Check sheet for the drawn part. Datum: minimum x, y, z corner. Units: mm. Round coordinates to 2 decimals unless told otherwise and drop trailing zeros. Order: outer loops, then holes, each group sorted by start corner. A loop starts at its lowest first (then second) coordinate and runs counter-clockwise, first axis right, second up.
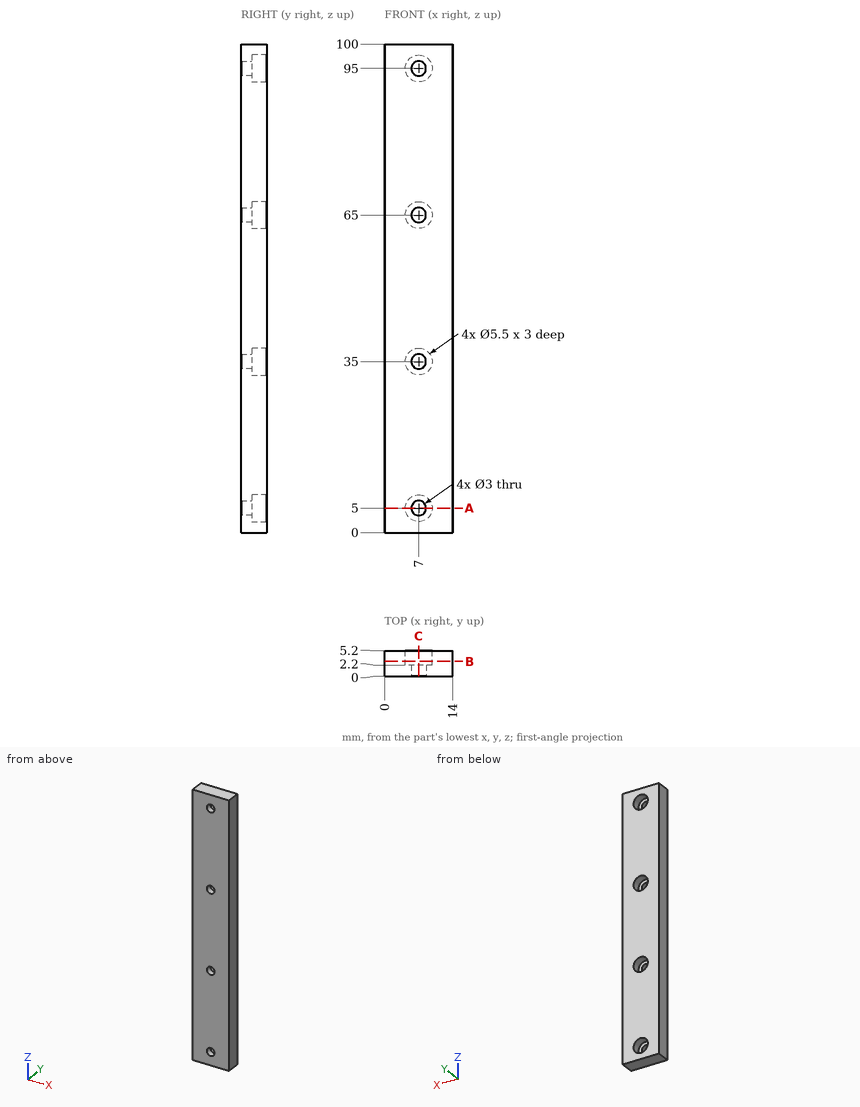
1) Sectioned sample at B-B on y = 3. Record the cut outline in (x, z), and give its area (3 significant figures).
2) Sectioned sample at C-C on x = 7. Count the separate pieces of the cut face and the enclosed holes in it, and give its area (3 significant figures).
3) Sectioned sample at A-A on z = 5. Record the cut outline in (x, y).
4) Gauge pin test, flat ends, axial feed: pin 1 (1.6 mm diameter, centred on x = 6, z = 36, fed in from +Y); pin 2 (2.5 mm diameter, centred on x = 7, z = 65, fed in from -Y). Record the tip position at first contact, or that the pin passes through.
5) Scan lines: line 1 (Z direction, x = 7, y = 0.8); line 2 (X direction, y = 0.5, z = 5); line 3 (Y direction, x = 8.5, z = 63). Record each from-to range of solid material in increasing order.
Values found:
1. outline: (0, 0) - (14, 0) - (14, 100) - (0, 100) - close; hole circle Ø5.5 at (7, 5); hole circle Ø5.5 at (7, 35); hole circle Ø5.5 at (7, 65); hole circle Ø5.5 at (7, 95)
1. area: 1,300 mm2
2. separate pieces: 5
2. enclosed holes: 0
2. area: 428 mm2
3. outline: (0, 0) - (5.5, 0) - (5.5, 2.2) - (4.25, 2.2) - (4.25, 5.2) - (0, 5.2) - close; (8.5, 0) - (14, 0) - (14, 5.2) - (9.75, 5.2) - (9.75, 2.2) - (8.5, 2.2) - close
4. pin 1: stops at y = 2.2
4. pin 2: passes through
5. line 1: z = 0 to 3.5, 6.5 to 33.5, 36.5 to 63.5, 66.5 to 93.5, 96.5 to 100
5. line 2: x = 0 to 5.5, 8.5 to 14
5. line 3: y = 0 to 2.2
